```python
from build123d import *

# Parameters (mm, degrees)
SKETCH1_R           = 5
SKETCH1_R_2         = 2.1
SKETCH1_W           = 5
SKETCH1_H           = 20
SKETCH1_W_2         = 8
SKETCH1_H_2         = 32
SKETCH1_W_3         = 3.5
SKETCH1_H_3         = 10
BOSS_EXTRUDE1_DEPTH = 5
CHAMFER1_SIZE       = 1
SKETCH3_R           = 1.435
BOSS_EXTRUDE2_DEPTH = 3.5


with BuildPart() as part:
    # Sketch1 → Boss-Extrude1 (new body)
    with BuildSketch(Plane(origin=(0, 0, 0), x_dir=(1, 0, 0), z_dir=(0, 1, 0))):
        Polygon((50, 16), (50, -41), (-50, -41), (-50, 41), (50, 41), (50, 36), align=None)
        with Locations(Location((40, -1.5, 0), (0, 0, 270))):
            Circle(SKETCH1_R, mode=Mode.SUBTRACT)
        with Locations(Location((-15.1, 14.5, 0), (0, 0, 270))):
            Circle(SKETCH1_R_2, mode=Mode.SUBTRACT)
        with Locations(Location((-15.1, -14.5, 0), (0, 0, 270))):
            Circle(SKETCH1_R_2, mode=Mode.SUBTRACT)
        with Locations((42.5, 26)):
            Rectangle(SKETCH1_W, SKETCH1_H, mode=Mode.SUBTRACT)
        with Locations((-33, 0)):
            Rectangle(SKETCH1_W_2, SKETCH1_H_2, mode=Mode.SUBTRACT)
        with Locations((-15.1, 0)):
            Rectangle(SKETCH1_W_3, SKETCH1_H_3, mode=Mode.SUBTRACT)
    extrude(amount=BOSS_EXTRUDE1_DEPTH)

    # Chamfer1
    chamfer1_edges = [part.edges().sort_by_distance(p)[0] for p in [
        (50, 5, 0),
        (0, 5, -41),
        (-50, 5, 0),
        (0, 5, 41),
    ]]
    chamfer(chamfer1_edges, length=CHAMFER1_SIZE)

    # Sketch3 → Boss-Extrude2 (add)
    with BuildSketch(Plane.XZ):
        with Locations(Location((47.5, 35, 0), (0, 0, 90))):
            Circle(SKETCH3_R)
        with Locations(Location((-47.5, 35, 0), (0, 0, 270))):
            Circle(SKETCH3_R)
        with Locations(Location((47.5, -35, 0), (0, 0, 270))):
            Circle(SKETCH3_R)
        with Locations(Location((-47.5, -35, 0), (0, 0, 90))):
            Circle(SKETCH3_R)
    extrude(amount=BOSS_EXTRUDE2_DEPTH)


solid = part.part
```
Work out the finished part from the listing and answer in its coordinate system (mm). A direction names the side the tool comes from. Give positions to 0.01 mm unless a question says otherwise; leave off trailing zeros. Loops run counter-clockwise (first coordinate to the right, second up) from the corner with the lowest first, then second, coordinate; pieces in that order, holes last. Notation, with made-up numbers: (47, 36.5) -> (63, 36.5) arc R28 cw to (63, 59.5) -> close; hole circle Ø2 at (-13.75, 59). An arc over 180 degrees is marked (long way). Write item = value, one per line. Start each with the question number.
(1) Given pin 1 Ø10 at (x, z) = (12, 14) entering from -Y; pin 2 Ø9 at (x, z) = (40, 1.5) entering from -Y, each flat-ended and moving along its own axis, determine where each tip first touches the part or whether it passes through.
(2) Find the intervals of material crossed by probe 1 along X at (y, z) = (1.5, 14.5); probe 2 along Z at (x, y) = (-35, 2.75); probe 3 along X at (y, z) = (0.75, -11), in increasing order. Write a range as from..to.
(3) Find section A-A on z = 1.5. Give the vertices of the cut face in (x, y), and give its area (4 significant figures).
(4) Find section B-B on z = 14.5. Give the vertices of the cut face in (x, y), and give its area (3 significant figures).
(5) Find section C-C on x = 17.5. Give the vertices of the cut face in (y, z), and give its area (3 significant figures).
(6) Find section D-D on y = -1.5. Give the vertices of the cut face in (x, z) (3 decimals).
(7) The mould has two halves that part along X. Classify faces 4 (the flat face through (42, 2, -16)), 5 (the flat face through (1, 2, 41)), 6 (the flat face through (-50, 2, 1)): +X half, -X half, draft (parallel to the pull), parting line (faces both ways), or undercut.
(8) Which of the six approach directions +Z, -Z, +X, -X, +Y, -Y give full straight-line access (tool end or side, diameter ignored) to faces 1 (the flat face through (-47, -3.5, 35)), 2 (the cylindrical face through (-48.773, -1.726, 34.338)), 3 (the flat face through (45, 2, -26))?
From the geometry:
q1.pin_1 = 0
q1.pin_2 = through
q2.probe_1 = -50..-37, -29..-17.2, -13..50
q2.probe_2 = -41..-16, 16..41
q2.probe_3 = -50..-37, -29..50
q3.outline = (-50, 0) -> (-37, 0) -> (-37, 5) -> (-49, 5) -> (-50, 4) -> close; (-29, 0) -> (-16.85, 0) -> (-16.85, 5) -> (-29, 5) -> close; (-13.35, 0) -> (35, 0) -> (35, 5) -> (-13.35, 5) -> close; (45, 0) -> (50, 0) -> (50, 4) -> (49, 5) -> (45, 5) -> close
q3.area = 391.5 mm^2
q4.outline = (-50, 0) -> (-37, 0) -> (-37, 5) -> (-49, 5) -> (-50, 4) -> close; (-29, 0) -> (-17.2, 0) -> (-17.2, 5) -> (-29, 5) -> close; (-13, 0) -> (50, 0) -> (50, 4) -> (49, 5) -> (-13, 5) -> close
q4.area = 438 mm^2
q5.outline = (0, -41) -> (4, -41) -> (5, -40) -> (5, 40) -> (4, 41) -> (0, 41) -> close
q5.area = 409 mm^2
q6.outline = circle Ø2.87 at (-47.5, -35); circle Ø2.87 at (-47.5, 35); circle Ø2.87 at (47.5, -35); circle Ø2.87 at (47.5, 35)
q7.face_4 = undercut
q7.face_5 = draft
q7.face_6 = -X half
q8.face_1 = +Z, -Z, +X, -X, -Y
q8.face_2 = -Y
q8.face_3 = +Y, -Y
